from build123d import *

# Parameters (mm, degrees)
SKETCH1_R           = 15
SKETCH1_R_2         = 2.4892
BOSS_EXTRUDE1_DEPTH = 4.7625


with BuildPart() as part:
    # Sketch1 → Boss-Extrude1 (new body)
    with BuildSketch(Plane(origin=(0, 0, 0), x_dir=(1, 0, 0), z_dir=(0, 1, 0))):
        with BuildLine():
            Line((-66.545030839, 29.74801255), (-78.71799706, 9.993951739))
            ThreePointArc((-78.71799706, 9.993951739), (-81.55, 0), (-78.71799706, -9.993951739))
            Line((-78.71799706, -9.993951739), (-66.545030839, -29.74801255))
            ThreePointArc((-66.545030839, -29.74801255), (-52.270546345, -35.304264568), (-43.033032799, -23.085378057))
            Line((-43.033032799, -23.085378057), (-43.033032799, 23.085378057))
            ThreePointArc((-43.033032799, 23.085378057), (-52.270546345, 35.304264568), (-66.545030839, 29.74801255))
        make_face()
        with Locations((-62.5, 0)):
            Circle(SKETCH1_R, mode=Mode.SUBTRACT)
        with Locations((-55.733032799, 23.085378057)):
            Circle(SKETCH1_R_2, mode=Mode.SUBTRACT)
        with Locations((-55.733032799, -23.085378057)):
            Circle(SKETCH1_R_2, mode=Mode.SUBTRACT)
    extrude(amount=BOSS_EXTRUDE1_DEPTH)


solid = part.part
Model file for the job. Use its own axes, mm. Give positions to 0.01 mm unless a question says otherwise; leave off trailing zeros. Loops run counter-clockwise (first coordinate to the right, second up) from the corner with the lowest first, then second, coordinate; pieces in that order, holes last.
1) Pull direction Z, two halves, no side cores. Call faces 1 (the flat face through (-72.546, 2.348, -20.009)), 2 (the cylindrical face through (-52.493, 2.348, 35.365)), 3 (the cylindrical face through (-77.485, 2.348, -0.66)), 4 (the flat face through (-49.7, 4.762, -8.5)): +Z half, -Z half, draft (parallel to the pull), parting line (faces both ways), or undercut.
2) Flat gauge pins, fed straight in: pin 1 Ø1.5 at (x, y) = (-72, 1) entering from +Z; pin 2 Ø3 at (x, z) = (-55.73, -23.09) entering from +Y. Where does each tip first touch, or does it go through?
3) Wall check: line 1 (X direction, y = 3.8, z = 0); line 2 (Z direction, x = -55.5, y = 2.65); line 3 (X direction, y = 2.75, z = 6.5). Give the ranges that are in metal, low to high.
4) Saw through at A-A (z = 0). Write the cut outline in (x, y), plus the area to 3 significant figures.
5) Saw through at B-B (x = -48.5). Write the cut outline in (y, z), plus the area to 3 significant figures.
6) Saw through at D-D (z = 17.5). Write the cut outline in (x, y), plus the area to 3 significant figures.
7) Saw through at C-C (y = 3.95). Write the cut outline in (x, z), plus the area to 3 significant figures.
Answer block:
1. face 1: -Z half
1. face 2: +Z half
1. face 3: undercut
1. face 4: draft
2. pin 1: stops at z = 22.11
2. pin 2: passes through
3. line 1: x = -81.55 to -77.5, -47.5 to -43.03
3. line 2: z = -35.78 to -25.56, -20.61 to -13.27, 13.27 to 20.61, 25.56 to 35.78
3. line 3: x = -80.41 to -76.02, -48.98 to -43.03
4. outline: (-81.55, 0) - (-77.5, 0) - (-77.5, 4.76) - (-81.55, 4.76) - close; (-47.5, 0) - (-43.03, 0) - (-43.03, 4.76) - (-47.5, 4.76) - close
4. area: 40.6 mm2
5. outline: (0, -33.52) - (4.76, -33.52) - (4.76, -5.39) - (0, -5.39) - close; (0, 5.39) - (4.76, 5.39) - (4.76, 33.52) - (0, 33.52) - close
5. area: 268 mm2
6. outline: (-74.09, 0) - (-43.03, 0) - (-43.03, 4.76) - (-74.09, 4.76) - close
6. area: 148 mm2
7. outline: (-78.72, -9.99) - (-66.55, -29.75) arc R12.7 ccw to (-43.03, -23.09) - (-43.03, 23.09) arc R12.7 ccw to (-66.55, 29.75) - (-78.72, 9.99) arc R19.05 ccw to start; hole circle Ø30 at (-62.5, 0); hole circle Ø4.98 at (-55.73, -23.09); hole circle Ø4.98 at (-55.73, 23.09)
7. area: 1,350 mm2
